Build history of the part. All positions in model axes, mm. Face numbers are marked on the shaded views. A direction names the side the tool comes from. Give positions to 0.01 mm unless a question says otherwise; leave off trailing zeros. Order: outer loops, then holes, each group sorted by start corner. A loop starts at its lowest first (then second) coordinate and runs counter-clockwise, first axis right, second up. Notation, with made-up numbers: (-27, 3.25) - (-18, 3.25) arc R15 ccw to (-18, 10.25) - close; hole circle Ø7 at (-33, 47.5). An arc over 180 degrees is marked (long way). One line per item, written item: value.
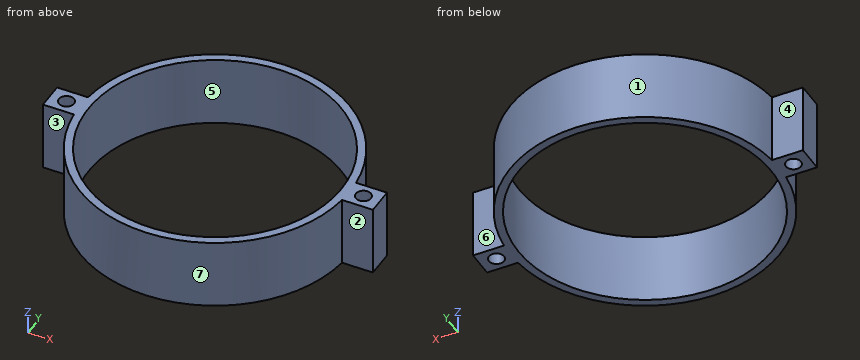
Autodesk Fusion 360 part; units mm, degrees
sketch "Sketch1" plane through (0, 0, 0) normal (0, 0, 1) x (1, 0, 0)
  circle A0 centre (0, 0) radius 42 construction
  line L0 (0, 0) -> (0, 42) construction
  circle A1 centre (0, 42) radius 2.25
  circle A2 centre (-17.0829, 38.3689) radius 2.25
  circle A3 centre (-31.2121, 28.1035) radius 2.25
  circle A4 centre (-39.9444, 12.9787) radius 2.25
  circle A5 centre (-41.7699, -4.3902) radius 2.25
  circle A6 centre (-36.3731, -21) radius 2.25
  circle A7 centre (-24.687, -33.9787) radius 2.25
  circle A8 centre (-8.7323, -41.0822) radius 2.25
  circle A9 centre (8.7323, -41.0822) radius 2.25
  circle A10 centre (24.687, -33.9787) radius 2.25
  circle A11 centre (36.3731, -21) radius 2.25
  circle A12 centre (41.7699, -4.3902) radius 2.25
  circle A13 centre (39.9444, 12.9787) radius 2.25
  circle A14 centre (31.2121, 28.1035) radius 2.25
  circle A15 centre (17.0829, 38.3689) radius 2.25
  circle A16 centre (0, 42) radius 3 construction
  circle A17 centre (-17.0829, 38.3689) radius 3 construction
  circle A18 centre (-31.2121, 28.1035) radius 3 construction
  circle A19 centre (-39.9444, 12.9787) radius 3 construction
  circle A20 centre (-41.7699, -4.3902) radius 3 construction
  circle A21 centre (-36.3731, -21) radius 3 construction
  circle A22 centre (-24.687, -33.9787) radius 3 construction
  circle A23 centre (-8.7323, -41.0822) radius 3 construction
  circle A24 centre (8.7323, -41.0822) radius 3 construction
  circle A25 centre (24.687, -33.9787) radius 3 construction
  circle A26 centre (36.3731, -21) radius 3 construction
  circle A27 centre (41.7699, -4.3902) radius 3 construction
  circle A28 centre (39.9444, 12.9787) radius 3 construction
  circle A29 centre (31.2121, 28.1035) radius 3 construction
  circle A30 centre (17.0829, 38.3689) radius 3 construction
  circle A31 centre (0, 0) radius 46
  circle A32 centre (0, 0) radius 49
  dimension "d1" = 84
  dimension "d2" = 4.5
  dimension "d4" = 360
  dimension "d5" = 6
  dimension "d7" = 360
  dimension "d8" = 92
  dimension "d9" = 3
extrude "Extrude1" add sketch "Sketch1" along normal blind 26 contours A32
sketch "Sketch2" plane through (0, 0, 26) normal (0, 0, 1) x (-1, 0, 0)
  circle A0 centre (0, 0) radius 46
  circle A1 centre (0, 0) radius 49
  line L0 (0, 0) -> (-69, 0) construction
  line L1 (0, 0) -> (0, -46) construction
  line L2 (-48.7442, -5) -> (-60, -5)
  line L3 (-60, -5) -> (-60, 5)
  line L4 (-60, 5) -> (-48.7442, 5)
  circle A2 centre (-54, 0) radius 2.75
  line L5 (48.7442, -5) -> (60, -5)
  line L6 (60, -5) -> (60, 5)
  line L7 (60, 5) -> (48.7442, 5)
  circle A3 centre (54, 0) radius 2.75
  dimension "d12" = 5.5
  dimension "d13" = 54
  dimension "d14" = 6
  dimension "d15" = 10
extrude "Extrude2" add sketch "Sketch2" against normal blind 26 contours A1 L5 L6 L7 | A1 L2 L3 L4
(1) Slice it at B-B, the plane z = 6.75. Give the cut face in (x, y), and give its area (3 significant figures).
Completed:
outline: (-60, -5) - (-48.74, -5) arc R49 ccw to (48.74, -5) - (60, -5) - (60, 5) - (48.74, 5) arc R49 ccw to (-48.74, 5) - (-60, 5) - close; hole circle Ø5.5 at (-54, 0); hole circle Ø92 at (0, 0); hole circle Ø5.5 at (54, 0)
area: 1,070 mm²
(2) Slice it at D-D, the plane y = 18. Give the cut face in (x, z).
Completed:
outline: (-45.57, 0) - (-42.33, 0) - (-42.33, 26) - (-45.57, 26) - close; (42.33, 0) - (45.57, 0) - (45.57, 26) - (42.33, 26) - close
(3) Pin check, flat tips, straight feed: P1, Ø4, axis at x = -29, z = 17.5, coming from the +Y side; P2, Ø3.5, axis at x = 54, y = 0, coming from the +Z side; P3, Ø9, axis at x = -56.5, z = 6.5, coming from the +Y side; P4, Ø5.5, axis at x = -56.5, z = 17, coming from the -Y side. Stop position of each tip, or through.
Completed:
P1: y = 40.89
P2: through
P3: y = 5
P4: y = -5
(4) 3-axis set-ups, long thin cutter, end or side, ignore diameter. For the marked faces 1, 2, 3 and 4: which of +Z, -Z, +X, -X, +Y, -Y reach the whole face in a straight line?
Completed:
face 1: +Z, -Z, +Y
face 2: +Z, -Z, +X, -Y
face 3: +Z, -Z, -X, -Y
face 4: +Z, -Z, -X, +Y
(5) Slice it at C-C, the plane y = 0. Give the cut face in (x, z).
Completed:
outline: (-60, 0) - (-56.75, 0) - (-56.75, 26) - (-60, 26) - close; (-51.25, 0) - (-46, 0) - (-46, 26) - (-51.25, 26) - close; (46, 0) - (51.25, 0) - (51.25, 26) - (46, 26) - close; (56.75, 0) - (60, 0) - (60, 26) - (56.75, 26) - close
(6) Slice it at A-A, the plane x = 54. Give the cut face in (y, z), and give its area (3 significant figures).
Completed:
outline: (-5, 0) - (-2.75, 0) - (-2.75, 26) - (-5, 26) - close; (2.75, 0) - (5, 0) - (5, 26) - (2.75, 26) - close
area: 117 mm²
(7) Pull direction X, two halves, no side cores. Call the marked faces 5, 6 and 7: +X half, -X half, draft (parallel to the pull), parting line (faces both ways), or undercut.
Completed:
face 5: undercut
face 6: draft
face 7: parting line
(8) Drill centre lines: line 1 (Y direction, x = 0, z = 9); line 2 (Y direction, x = -54, z = 6.25); line 3 (X direction, y = -36, z = 11.25). Where is each one in solid material? Low to high.
Completed:
line 1: -49 to -46, 46 to 49
line 2: -5 to -2.75, 2.75 to 5
line 3: -33.24 to -28.64, 28.64 to 33.24
